Geometry: final body of the model. Coordinates: model frame, mm. A direction names the side the tool comes from. Give positions to 0.01 mm unless a question says otherwise; leave off trailing zeros. Write each loop counter-clockwise with the first axis right and the second up, starting at its lowest first coordinate (ties: lowest second). Pieces come first, ordered by that corner, then holes. Notation, with made-up numbers: (58.25, -17) - (98.25, -17) arc R21 cw to (98.25, 2) - close; hole circle Ø11 at (32.5, 72.5). An arc over 180 degrees is marked (long way). One line per question, with ' | ' between items. Start each with the question number.
Autodesk Inventor part; units mm, degrees
ref_plane "YZ Plane" through (0, 0, 0) normal (1, 0, 0) x (0, 1, 0)
ref_plane "XZ Plane" through (0, 0, 0) normal (0, 1, 0) x (-1, 0, 0)
ref_plane "XY Plane" through (0, 0, 0) normal (0, 0, 1) x (1, 0, 0)
sketch "Sketch1" plane through (0, 0, 0) normal (0, 0, 1) x (1, 0, 0)
  line L0 (-25, 0) -> (25, 0)
  line L1 (25, 0) -> (25, 29)
  line L2 (25, 29) -> (15, 29)
  line L3 (15, 29) -> (15, 36)
  line L4 (15, 36) -> (-15, 36)
  line L5 (-15, 36) -> (-15, 29)
  line L6 (-15, 29) -> (-25, 29)
  line L7 (-25, 29) -> (-25, 0)
  point P0 (0, 0)
  point P1 (0, 0)
  dimension "d0" = 50
  dimension "d1" = 36
  dimension "d2" = 7
  dimension "d3" = 30
extrude "Extrusion1" add sketch "Sketch1" along normal mid plane 22
sketch "Sketch2" plane through (0, 0, 11) normal (0, 0, 1) x (1, 0, 0)
  line L0 (-25, 0) -> (25, 0)
  point P0 (0, 0)
  point P1 (0, 21)
  point P2 (0, 0)
  dimension "d6" = 21
hole "Hole1" at (0, 21, 11) direction (0, 0, -1) diameter 22 end through all
chamfer "Chamfer2" distance 2 angle 45 2 edges at (-15, 36, 0) (15, 36, 0)
sketch "Sketch3" plane through (-25, 29, 11) normal (0, 1, 0) x (1, 0, 0)
  line L0 (0, 22) -> (0, 0)
  line L1 (50, 22) -> (50, 0)
  line L2 (50, 22) -> (0, 22)
  line L3 (0, 0) -> (50, 0)
  point P0 (25, 11)
  point P1 (6, 17)
  point P2 (44, 17)
  point P3 (6, 5)
  point P4 (44, 5)
  dimension "d20" = 38
  dimension "d21" = 6
  dimension "d22" = 6
  dimension "d49" = 12
  dimension "d50" = 5
  dimension "d51" = 5
hole "Hole2" at (-19, 29, -6) at (19, 29, -6) at (-19, 29, 6) at (19, 29, 6) direction (0, -1, 0) diameter 4.5 end through all counterbore diameter 8 counterbore depth 5
sketch "Sketch5" plane through (0, 0, 11) normal (0, 0, 1) x (1, 0, 0)
  circle A0 centre (0, 21) radius 11
  point P0 (0, 0)
  point P1 (-15, 21)
  point P2 (15, 21)
  dimension "d40" = 30
  dimension "d52" = 15
hole "Hole4" at (-15, 21, 11) at (15, 21, 11) direction (0, 0, -1) diameter 2.459 depth 10 tip angle 118
hole "Hole5" at (0, 21, -11) direction (0, 0, 1) diameter 26 depth 17.5
sketch "Sketch6" plane through (0, 0, -11) normal (0, 0, -1) x (-1, 0, 0)
  circle A0 centre (0, 21) radius 15.5563 construction
  circle A1 centre (0, 21) radius 13 construction
  point P0 (0, 0)
  point P1 (-11, 32)
  point P2 (-11, 10)
  point P3 (11, 10)
  point P4 (11, 32)
  dimension "d62" = 22
  dimension "d63" = 22
hole "Hole6" at (11, 32, -11) at (11, 10, -11) at (-11, 10, -11) at (-11, 32, -11) direction (0, 0, 1) diameter 2.459 depth 8 tip angle 118
properties part number "Lagerbock_Loslager" material "Aluminum 6061"
1) Reachability of faces 4 (the cylindrical face through (15.034, 26.465, 5.479)), 5 (the cylindrical face through (13.963, 20.339, 5.93)), 6 (the cylindrical face through (-3.9, 33.4, -2.1)) from +Z, -Z, +X, -X, +Y, -Y: full face, straight path, thin tool, end or side. Return the list, or none.
2) Pull-direction query (Y, two-part tool) for faces 1 (the conical face through (15.14, 21.16, 0.39)), 2 (the cylindrical face through (15.034, 26.465, -6.521)), 3 (the flat face through (-17, 24, -4)); classes: +Y half, -Y half, draft (parallel to the pull), parting line (faces both ways), or undercut.
3) Section B-B, the plane x = 19. Output: boundary loops of the cut face in (y, z), plus the area to 3 significant figures.
4) First-contact query: pin 1 Ø1.5 at (x, z) = (-1.5, -5) entering from -Y; pin 2 Ø3.5 at (x, z) = (19, -6) entering from -Y; pin 3 Ø6.5 at (x, z) = (19, -5) entering from +Y; pin 4 Ø9 at (x, z) = (-19, 6) entering from +Y. Flat tips, straight axial feed; report the tip coordinate or a pass-through.
5) Section C-C, the plane y = 18.5. Output: boundary loops of the cut face in (x, z), plus the area to 3 significant figures.
6) Line query: L1, parallel to X at y = 21, z = 8.5; L2, parallel to Z at x = -19.5, y = 14.5; L3, parallel to Y at x = 0, z = -7. Output: solid intervals per line, ascending.
7) Section D-D, the plane z = 9. Output: boundary loops of the cut face in (x, y).
8) Section A-A, the plane x = 0. Output: boundary loops of the cut face in (y, z).
Answer key:
1) face 4: +Y | face 5: +Z | face 6: -Z
2) face 1: undercut | face 2: draft | face 3: +Y half
3) outline: (0, -11) - (29, -11) - (29, -10) - (24, -10) - (24, -8.25) - (0, -8.25) - close; (0, -3.75) - (24, -3.75) - (24, -2) - (29, -2) - (29, 2) - (24, 2) - (24, 3.75) - (0, 3.75) - close; (0, 8.25) - (24, 8.25) - (24, 10) - (29, 10) - (29, 11) - (0, 11) - close | area: 342 mm^2
4) pin 1: y = 0 | pin 2: through | pin 3: y = 29 | pin 4: y = 34.5
5) outline: (-25, -11) - (-12.76, -11) - (-12.76, 6.5) - (-10.71, 6.5) - (-10.71, 11) - (-25, 11) - close; (10.71, 6.5) - (12.76, 6.5) - (12.76, -11) - (25, -11) - (25, 11) - (10.71, 11) - close; hole circle Ø4.5 at (-19, -6); hole circle Ø4.5 at (-19, 6); hole circle Ø4.5 at (19, -6); hole circle Ø4.5 at (19, 6) | area: 493 mm^2
6) L1: -25 to -16.23, -13.77 to -11, 11 to 13.77, 16.23 to 25 | L2: -11 to -8.19, -3.81 to 3.81, 8.19 to 11 | L3: 0 to 8, 34 to 36
7) outline: (-25, 0) - (25, 0) - (25, 29) - (21.65, 29) - (21.65, 24) - (16.35, 24) - (16.35, 29) - (15, 29) - (15, 34) - (13, 36) - (-13, 36) - (-15, 34) - (-15, 29) - (-16.35, 29) - (-16.35, 24) - (-21.65, 24) - (-21.65, 29) - (-25, 29) - close; hole circle Ø2.46 at (-15, 21); hole circle Ø22 at (0, 21); hole circle Ø2.46 at (15, 21)
8) outline: (0, -11) - (8, -11) - (8, 6.5) - (10, 6.5) - (10, 11) - (0, 11) - close; (32, 6.5) - (34, 6.5) - (34, -11) - (36, -11) - (36, 11) - (32, 11) - close
